Build history of the part. All positions in model axes, mm. Face numbers are marked on the shaded views. A direction names the side the tool comes from. Give positions to 0.01 mm unless a question says otherwise; leave off trailing zeros. Order: outer loops, then holes, each group sorted by start corner. A loop starts at its lowest first (then second) coordinate and runs counter-clockwise, first axis right, second up. Notation, with made-up numbers: (56.5, -16) - (88.5, -16) arc R14 cw to (88.5, -1) - close; hole circle Ø1 at (4, -40). An arc over 180 degrees is marked (long way). Write each question's results on one line, items separated by ' | '. Start each with the question number.
from build123d import *

# Parameters (mm, degrees)
CORTAR_EXTRUIR1_DEPTH = 3
CHAFL_N1_SIZE         = 0.5
REDONDEO1_R           = 0.5


with BuildPart() as part:
    # Croquis1 → Revolución1 (revolve)
    with BuildSketch(Plane.XY):
        Polygon((0, 0), (3.5, 0), (3.5, -4), (2, -4), (2, -16), (0, -16), align=None)
    revolve(axis=Axis((0, 0, 0), (0, -1, 0)))

    # Croquis2 → Cortar-Extruir1 (cut)
    with BuildSketch(Plane(origin=(0, 0, 0), x_dir=(1, 0, 0), z_dir=(0, 1, 0))):
        Polygon((1.5, 0.866025404), (0, 1.732050808), (-1.5, 0.866025404), (-1.5, -0.866025404), (0, -1.732050808), (1.5, -0.866025404), align=None)
    extrude(amount=-CORTAR_EXTRUIR1_DEPTH, mode=Mode.SUBTRACT)

    # Chaflán1
    chafl_n1_edges = [part.edges().sort_by_distance(p)[0] for p in [
        (-2, -16, 0),
    ]]
    chamfer(chafl_n1_edges, length=CHAFL_N1_SIZE)

    # Redondeo1
    redondeo1_edges = [part.edges().sort_by_distance(p)[0] for p in [
        (-3.5, 0, 0),
    ]]
    fillet(redondeo1_edges, radius=REDONDEO1_R)


solid = part.part
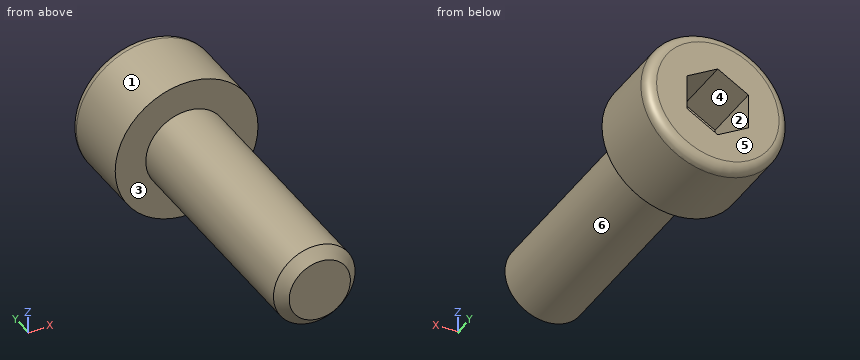
Item 1: Cut at C-C, the plane y = -3.5. List the corners of the cut face in (x, z).
Item 2: Flat gauge pins, fed straight in: pin 1 Ø1.5 at (y, z) = (-11.5, 2) entering from +X; pin 2 Ø1.5 at (x, z) = (0, 0) entering from +Y; pin 3 Ø4 at (x, y) = (-2.5, -2) entering from -Z. Where does each tip first touch, or does it go through?
Item 3: Cut at B-B, the plane z = 0. List the corners of the cut face in (x, y), then the cut area to 3 significant figures.
Item 4: Which spindle directions (+Z, -Z, +X, -X, +Y, -Y) get a long thin tool onto all of the face, cutting with end or side? Do the marked faces 1, 2 and 3. Say none if no direction does.
Item 5: Two-plate mould, pull along Z, no slides. Class the marked faces 4, 5 and 6: +Z half, -Z half, draft (parallel to the pull), parting line (faces both ways), or undercut.
Item 6: Cut at D-D, the plane y = -8. List the corners of the cut face in (x, z), then the cut area to 3 significant figures.
Item 7: Cut at A-A, the plane y = -1.75. List the corners of the cut face in (x, z), then the cut area to 3 significant figures.
Item 8: Probe line 1 along Y through (x, z) = (-1.75, -2.5); line 2 along X through (y, z) = (-0.5, 1.5); line 3 along Z through (x, y) = (-1, -1). List the from-to ranges inside material, lowest first. Write a range as from..to.
Values found:
1) outline: circle Ø7 at (0, 0)
2) pin 1: stops at x = 1.56 | pin 2: stops at y = -3 | pin 3: stops at z = -3.46
3) outline: (-3.5, -4) - (-2, -4) - (-2, -15.5) - (-1.5, -16) - (1.5, -16) - (2, -15.5) - (2, -4) - (3.5, -4) - (3.5, -0.5) arc R0.5 ccw to (3, 0) - (1.5, 0) - (1.5, -3) - (-1.5, -3) - (-1.5, 0) - (-3, 0) arc R0.5 ccw to (-3.5, -0.5) - close | area: 66.6 mm2
4) face 1: +Y, -Y | face 2: +Y | face 3: -Y
5) face 4: undercut | face 5: draft | face 6: parting line
6) outline: circle Ø4 at (0, 0) | area: 12.6 mm2
7) outline: circle Ø7 at (0, 0); hole (-1.5, -0.87) - (0, -1.73) - (1.5, -0.87) - (1.5, 0.87) - (0, 1.73) - (-1.5, 0.87) - close | area: 30.7 mm2
8) line 1: y = -4..0 | line 2: x = -3.16..-0.4, 0.4..3.16 | line 3: z = -3.35..-1.15, 1.15..3.35
